Study the drawing (mm; zero at the part's minimum x, y, z) and answer. Give positions to 0.01 mm unless a question says otherwise; leave off trailing zeros. Order: outer loops, then holes, each group sorted by start corner. A loop starts at its lowest first (then second) coordinate and runs counter-clockwise, first axis right, second up. Notation, with made-up numbers: (36, 57) - (95, 57) arc R10 cw to (95, 75) - close; hole circle Ø3 at (39.5, 88). An arc over 180 degrees is marked (long way). Put each result on its own line as item: value.
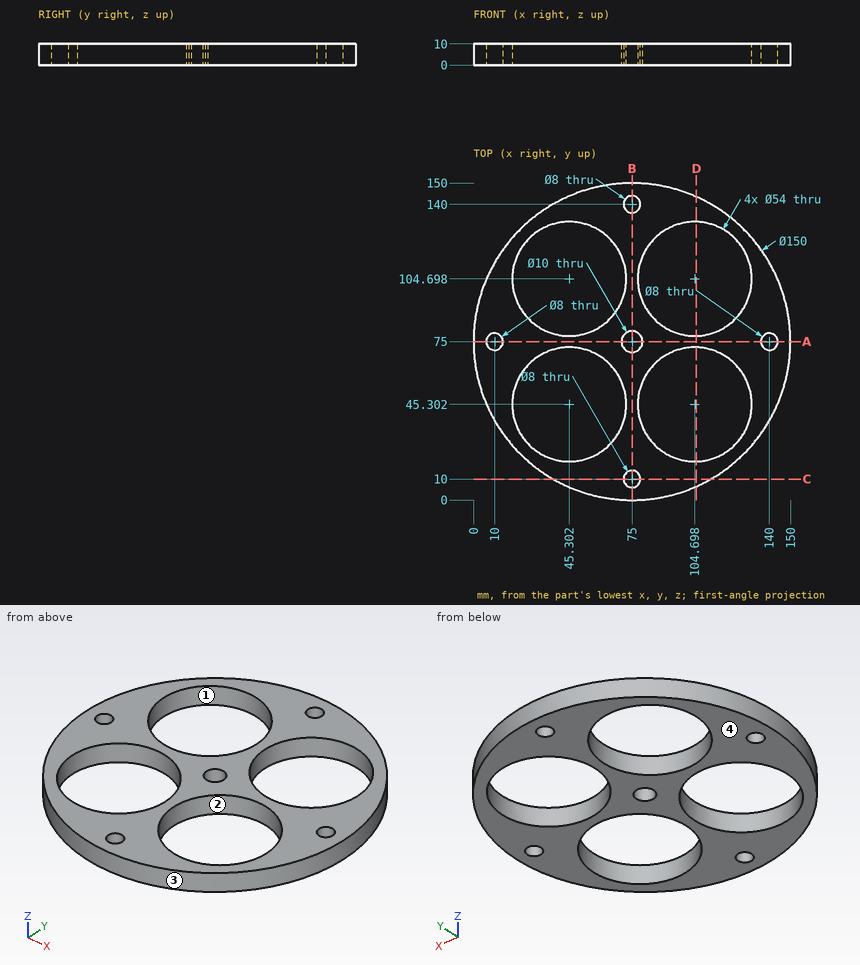
(1) Section C-C, the plane y = 10 is taken. Write down the section's boundary in (x, z).
Geometry check:
outline: (37.58, 0) - (71, 0) - (71, 10) - (37.58, 10) - close; (79, 0) - (112.42, 0) - (112.42, 10) - (79, 10) - close
(2) Straight lines are drawn through the part: line 1 (Y direction, x = 75, z = 8); line 2 (Y direction, x = 28.5, z = 2.75) (1 decimal); line 3 (Y direction, x = 97.5, z = 5.25) (1 decimal). For each, find the intervals that lie inside material, in ascending order.
Geometry check:
line 1: y = 0 to 6, 14 to 70, 80 to 136, 144 to 150
line 2: y = 16.2 to 24.2, 66.4 to 83.6, 125.8 to 133.8
line 3: y = 3.5 to 19.3, 71.3 to 78.7, 130.7 to 146.5
(3) Determine the mould class of the marked faces 1, 2, 3 and 4 for opening direction Y: pulls with the +Y half, pulls with the -Y half, needs draft (parallel to the pull), parting line crosses it, or undercut.
Geometry check:
face 1: undercut
face 2: undercut
face 3: parting line crosses it
face 4: needs draft
(4) Section D-D, the plane x = 105.5 is taken. Write down the section's boundary in (y, z), then the cut area to 3 significant figures.
Geometry check:
outline: (6.48, 0) - (18.31, 0) - (18.31, 10) - (6.48, 10) - close; (72.29, 0) - (77.71, 0) - (77.71, 10) - (72.29, 10) - close; (131.69, 0) - (143.52, 0) - (143.52, 10) - (131.69, 10) - close
area: 291 mm²
(5) Section A-A, the plane y = 75 is taken. Write down the section's boundary in (x, z), then the cut area to 3 significant figures.
Geometry check:
outline: (0, 0) - (6, 0) - (6, 10) - (0, 10) - close; (14, 0) - (70, 0) - (70, 10) - (14, 10) - close; (80, 0) - (136, 0) - (136, 10) - (80, 10) - close; (144, 0) - (150, 0) - (150, 10) - (144, 10) - close
area: 1,240 mm²
(6) Given pin 1 (1.5 mm diameter, centred on y = 63, z = 9, fed in from +X); pin 2 (5 mm diameter, centred on x = 75, y = 140, fed in from +Z); pin 3 (5 mm diameter, centred on x = 95.5, z = 3.5, fed in from +Y); pin 4 (13 mm diameter, centred on x = 10, y = 75, fed in from -Z), each flat-ended and moving along its own axis, determine where each tip first touches the part or whether it passes through.
Geometry check:
pin 1: stops at x = 149.15
pin 2: passes through
pin 3: stops at y = 147.81
pin 4: stops at z = 0
